Geometry check sheet. Reference: the model listing, model coordinates, mm. Round coordinates to 2 decimals unless told otherwise and drop trailing zeros. Write each loop counter-clockwise with the first axis right and the second up, starting at its lowest first coordinate (ties: lowest second). Pieces come first, ordered by that corner, then holes.
from build123d import *

# Parameters (mm, degrees)
F1_DEPTH = 1200
F3_D     = 5
F4_R     = 2


# Not quite as in the source:
# - a feature names something its author has since deleted; it is built from what else it names


with BuildPart() as f1:
    # F0 (on Right) → F1 (new body)
    with BuildSketch(Plane.YZ):
        Polygon((-18.8378913403, 177.8021101952), (-18.8378913403, 154.8021101952), (-16.8378913403, 154.8021101952), (-16.8378913403, 179.8021101952), (-56.8378913403, 179.8021101952), (-56.8378913403, 79.8021101952), (-29.8378913403, 79.8021101952), (-29.8378913403, 53.8021101952), (-27.8378913403, 53.8021101952), (-27.8378913403, 81.8021101952), (-54.8378913403, 81.8021101952), (-54.8378913403, 177.8021101952), align=None)
    extrude(amount=F1_DEPTH)

    # F3 (through all)
    with Locations(Plane.XZ.offset(29.8378913403)):
        with Locations((433, 66.8021101952), (767, 66.8021101952), (1100, 66.8021101952), (100, 66.8021101952)):
            Hole(F3_D / 2)

    # F4
    f4_edges = [f1.edges().sort_by_distance(p)[0] for p in [
        (600, -56.837891, 179.80211),
        (600, -16.837891, 179.80211),
        (600, -56.837891, 79.80211),
        (600, -27.837891, 81.80211),
        (600, -54.837891, 81.80211),
        (600, -29.837891, 79.80211),
        (600, -18.837891, 177.80211),
        (600, -54.837891, 177.80211),
    ]]
    fillet(f4_edges, radius=F4_R)


solid = f1.part
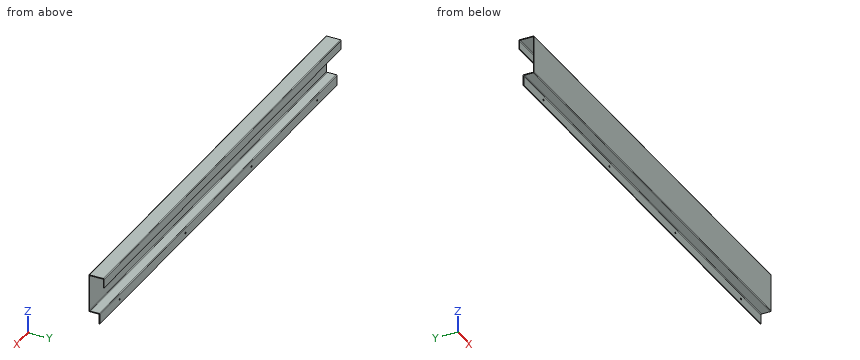
1. Section check C-C (z = 126.5). Record the cut outline in (x, y).
2. Section check A-A (y = -38.5). Record the cut outline in (x, z), plus the area to 3 significant figures.
3. Section check B-B (x = 370). Record the cut outline in (y, z), plus the area to 3 significant figures.
4. Depth check by flat-ended pin: pin 1 Ø1 at (x, y) = (816, -18) entering from -Z; pin 2 Ø4.5 at (x, z) = (100, 66.8) entering from -Y; pin 3 Ø6.5 at (x, z) = (767, 66.8) entering from +Y; pin 4 Ø4 at (x, z) = (858, 93) entering from +Y. Enter the tip coordinate at first touch or a pass-through.
5. Scan lines: line 1 along Z through (x, y) = (767, -29); line 2 along Z through (x, y) = (767, -28.55); line 3 along Z through (x, y) = (734, -43.5). Record each from-to range of solid material in increasing order.
Results below:
1. outline: (0, -56.84) - (1200, -56.84) - (1200, -54.84) - (0, -54.84) - close
2. outline: (0, 79.8) - (1200, 79.8) - (1200, 81.8) - (0, 81.8) - close; (0, 177.8) - (1200, 177.8) - (1200, 179.8) - (0, 179.8) - close
2. area: 4,800 mm2
3. outline: (-56.84, 81.8) arc R2 ccw to (-54.84, 79.8) - (-31.84, 79.8) arc R2 cw to (-29.84, 77.8) - (-29.84, 53.8) - (-27.84, 53.8) - (-27.84, 79.8) arc R2 ccw to (-29.84, 81.8) - (-52.84, 81.8) arc R2 cw to (-54.84, 83.8) - (-54.84, 175.8) arc R2 cw to (-52.84, 177.8) - (-20.84, 177.8) arc R2 cw to (-18.84, 175.8) - (-18.84, 154.8) - (-16.84, 154.8) - (-16.84, 177.8) arc R2 ccw to (-18.84, 179.8) - (-54.84, 179.8) arc R2 ccw to (-56.84, 177.8) - close
3. area: 428 mm2
4. pin 1: stops at z = 154.8
4. pin 2: passes through
4. pin 3: stops at y = -27.84
4. pin 4: stops at y = -54.84
5. line 1: z = 53.8 to 64.3, 69.3 to 81.62, 177.8 to 179.8
5. line 2: z = 53.8 to 64.3, 69.3 to 81.33, 177.8 to 179.8
5. line 3: z = 79.8 to 81.8, 177.8 to 179.8
